Study the drawing (mm; zero at the part's minimum x, y, z) and answer. Round coordinates to 2 decimals unless told otherwise and drop trailing zeros. Loops run counter-clockwise (first coordinate to the right, second up) from the corner with the lowest first, then second, coordinate; pieces in that order, holes last. Notation, with made-up numbers: M 37,25.5 L 56,25.5 A21 cw 56,45.5 Z; hole C 41,34 d10. An arc over 180 degrees is marked long. Write each question's results on one line, items separated by ' | '.
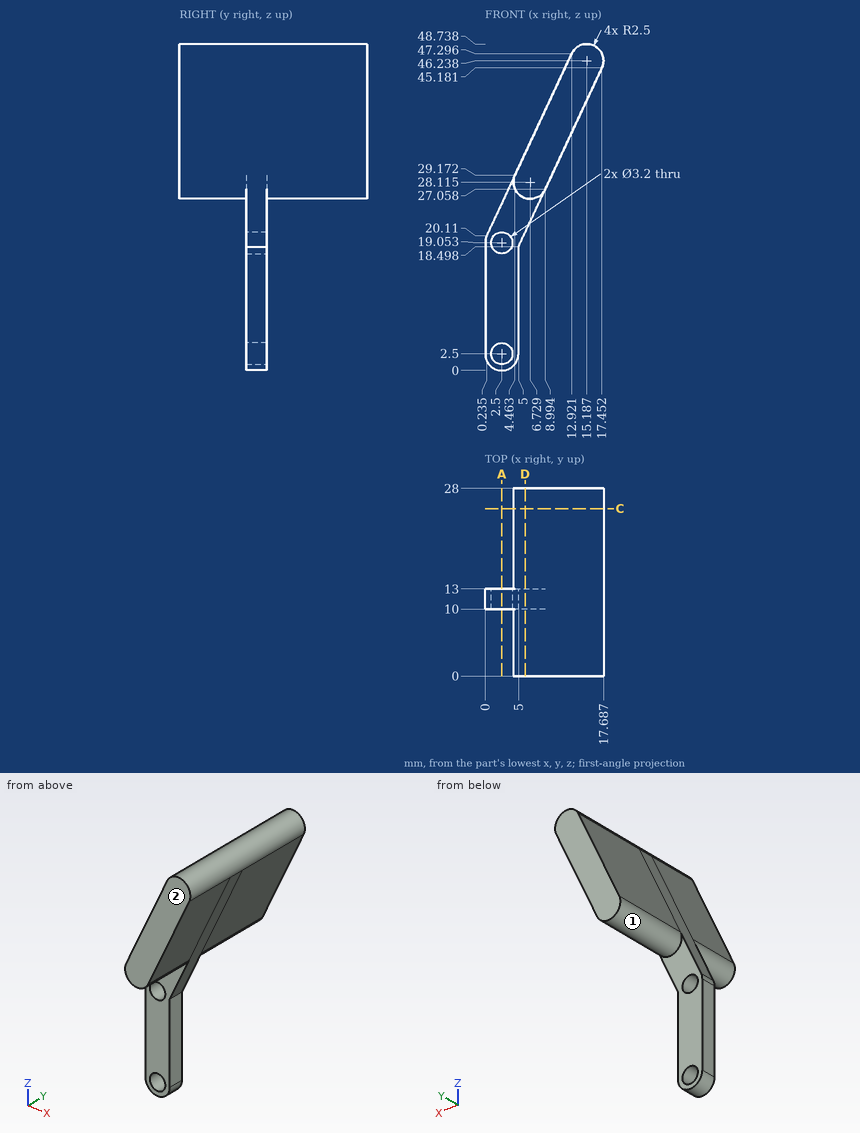
Item 1: The part is cut by section C-C (y = 25). Determine the outline of the cut face in (x, z) (1 decimal).
Outcome:
outline: M 4.5,29.2 A2.5 ccw 9,27.1 L 17.5,45.2 A2.5 ccw 12.9,47.3 Z
Item 2: The mould has two halves that part along Z. Classify the marked faces 1 and 2: pulls with the +Z half, pulls with the -Z half, needs draft (parallel to the pull), parting line crosses it, or undercut.
Outcome:
face 1: parting line crosses it | face 2: needs draft
Item 3: Flat-ended cylindrical pins translate along their axes: pin 1 (4 mm diameter, centred on x = 10, y = 11.5, fed in from -Z) (1 decimal); pin 2 (2.5 mm diameter, centred on x = 3.5, z = 21.5, fed in from +Y); pin 3 (5 mm diameter, centred on x = 13.5, y = 20.5, fed in from -Z) (1 decimal); pin 4 (3 mm diameter, centred on x = 2.5, z = 2.5, fed in from +Y). Find the tip coordinate at first contact, or state that the pin passes through.
Outcome:
pin 1: stops at z = 24.9 | pin 2: stops at y = 13 | pin 3: stops at z = 31.4 | pin 4: passes through
Item 4: The part is cut by section A-A (x = 2.5). Determine the outline of the cut face in (y, z) (1 decimal).
Outcome:
outline: M 10,0 L 13,0 L 13,0.9 L 10,0.9 Z; M 10,4.1 L 13,4.1 L 13,17.5 L 10,17.5 Z; M 10,20.7 L 13,20.7 L 13,25 L 10,25 Z
Item 5: The part is cut by section D-D (x = 6). Determine the outline of the cut face in (y, z) (1 decimal), plus the area to 3 significant figures.
Outcome:
outline: M 0,25.7 L 10,25.7 L 10,20.6 L 13,20.6 L 13,25.7 L 28,25.7 L 28,32.5 L 0,32.5 Z | area: 204 mm2
Item 6: Straight lines are drawn through the part: line 1 (X direction, y = 11.2, z = 2.5); line 2 (X direction, y = 4.25, z = 26) (1 decimal); line 3 (Z direction, x = 11.75, y = 8) (1 decimal). For each, find the intervals that lie inside material, in ascending order.
Outcome:
line 1: x = 0 to 0.9, 4.1 to 5 | line 2: x = 5.4 to 8.1 | line 3: z = 33 to 44.8
